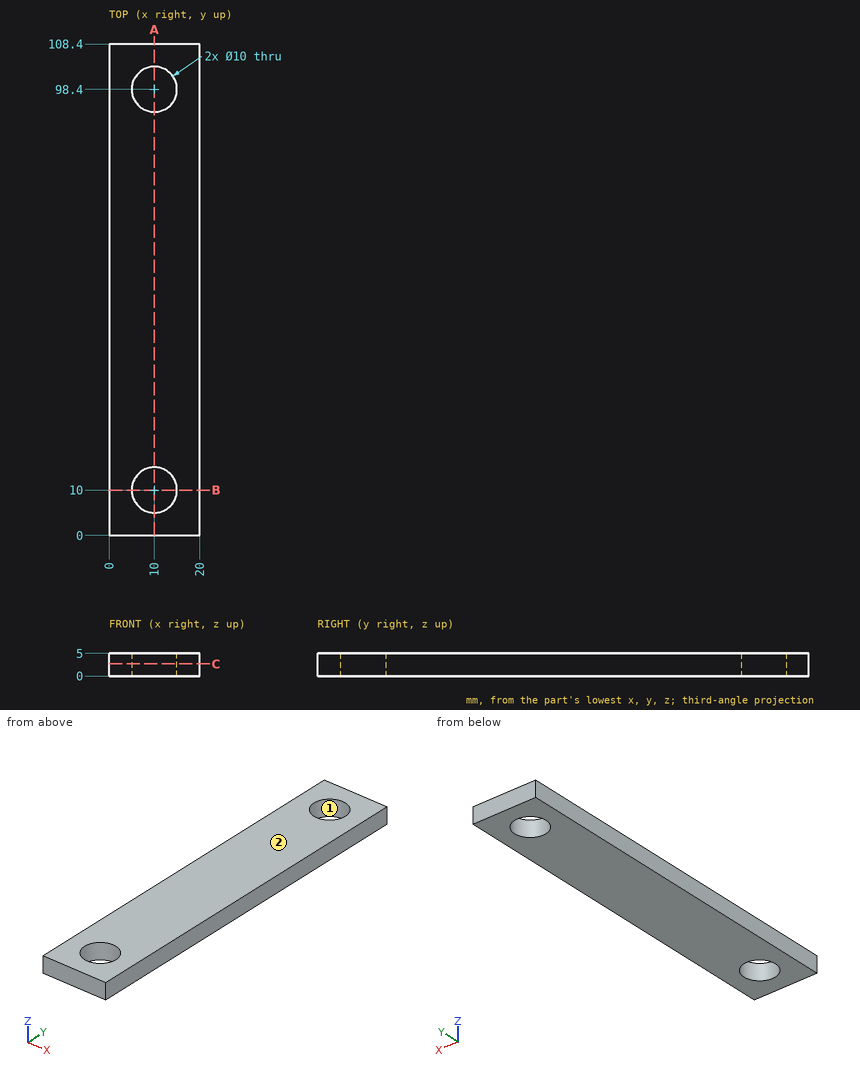
Input: dimensioned drawing with shaded views. Units: mm. Origin: part minimum x, y, z. Coordinates: 2 decimals unless noted, no trailing zeros. Order: outer loops, then holes, each group sorted by start corner. A loop starts at its lowest first (then second) coordinate and runs counter-clockwise, first axis right, second up. Notation, with made-up numbers: (-22, 7.25) -> (5, 7.25) arc R19 cw to (5, 23.25) -> close; hole circle Ø7 at (53, 46). An arc over 180 degrees is marked (long way). Answer in a Markdown table with one row per item.
Item 1: Section C-C on z = 2.7. Output: boundary loops of the cut face in (x, y), plus the area to 3 significant figures.
Return value:
| item | result |
|---|---|
| outline | (0, 0) -> (20, 0) -> (20, 108.4) -> (0, 108.4) -> close; hole circle Ø10 at (10, 10); hole circle Ø10 at (10, 98.4) |
| area | 2,010 mm² |
Item 2: Section B-B on y = 10. Output: boundary loops of the cut face in (x, z).
Return value:
| item | result |
|---|---|
| outline | (0, 0) -> (5, 0) -> (5, 5) -> (0, 5) -> close; (15, 0) -> (20, 0) -> (20, 5) -> (15, 5) -> close |
Item 3: Draft query along Y for the marked faces 1 and 2. Return one class per face: released by +Y, released by -Y, zero draft, split by the parting line, or undercut.
Return value:
| item | result |
|---|---|
| face 1 | undercut |
| face 2 | zero draft |
Item 4: Ray query, L1, parallel to Y at x = 10, z = 1.75; L2, parallel to Y at x = 8, z = 2.45; L3, parallel to X at y = 12.5, z = 3.95. Return the intervals inside material, ascending.
Return value:
| item | result |
|---|---|
| L1 | y = 0 to 5, 15 to 93.4, 103.4 to 108.4 |
| L2 | y = 0 to 5.42, 14.58 to 93.82, 102.98 to 108.4 |
| L3 | x = 0 to 5.67, 14.33 to 20 |
Item 5: Section A-A on x = 10. Output: boundary loops of the cut face in (y, z), plus the area to 3 significant figures.
Return value:
| item | result |
|---|---|
| outline | (0, 0) -> (5, 0) -> (5, 5) -> (0, 5) -> close; (15, 0) -> (93.4, 0) -> (93.4, 5) -> (15, 5) -> close; (103.4, 0) -> (108.4, 0) -> (108.4, 5) -> (103.4, 5) -> close |
| area | 442 mm² |
